```python
from build123d import *

# Parameters (mm, degrees)
SKETCH1_R           = 250
BOSS_EXTRUDE1_DEPTH = 5
SKETCH5_OUTSIDE_W   = 643.424
SKETCH5_OUTSIDE_H   = 643.424
CUT_EXTRUDE4_DEPTH  = 6
SKETCH6_R           = 2
CUT_EXTRUDE5_DEPTH  = 346.046056454
CUT_EXTRUDE6_DEPTH  = 346.046056454
SKETCH8_W           = 94.99
SKETCH8_H           = 32
CUT_EXTRUDE7_DEPTH  = 346.046056454
CUT_EXTRUDE8_DEPTH  = 346.046056454
FILLET1_R           = 2


with BuildPart() as part:
    # Sketch1 → Boss-Extrude1 (new body)
    with BuildSketch(Plane(origin=(0, 0, 0), x_dir=(1, 0, 0), z_dir=(0, 1, 0))):
        with Locations(Location((0, 0, 0), (0, 0, 270))):
            Circle(SKETCH1_R)
    extrude(amount=BOSS_EXTRUDE1_DEPTH)

    # Sketch5 outside → Cut-Extrude4 (cut)
    with BuildSketch(Plane(origin=(0, 5, 0), x_dir=(1, 0, 0), z_dir=(0, 1, 0))):
        Rectangle(SKETCH5_OUTSIDE_W, SKETCH5_OUTSIDE_H)
        Polygon((-139.754248594, -192.355221073), (139.754248594, -192.355221073), (202.254248594, -146.946313073), (250, 0), (202.254248594, 146.946313073), (77.254248594, 237.764129074), (-77.254248594, 237.764129074), (-202.254248594, 146.946313073), (-250, 0), (-202.254248594, -146.946313073), align=None, mode=Mode.SUBTRACT)
    extrude(amount=-CUT_EXTRUDE4_DEPTH, mode=Mode.SUBTRACT)

    # Sketch6 → Cut-Extrude5 (cut, through all)
    with BuildSketch(Plane.XZ):
        with Locations(Location((-3.899248594, 181.855221073, 0), (0, 0, 270))):
            Circle(SKETCH6_R)
        with Locations(Location((-199.656287114, 120.963302587, 0), (0, 0, 270))):
            Circle(SKETCH6_R)
        with Locations(Location((-232.625774638, -19.493653604, 0), (0, 0, 270))):
            Circle(SKETCH6_R)
        with Locations(Location((-176.74012291, -152.504696683, 0), (0, 0, 270))):
            Circle(SKETCH6_R)
        with Locations(Location((-53.345751406, -227.264129074, 0), (0, 0, 270))):
            Circle(SKETCH6_R)
        with Locations(Location((90.424883979, -215.216388582, 0), (0, 0, 270))):
            Circle(SKETCH6_R)
        with Locations(Location((199.656287114, -120.963302587, 0), (0, 0, 270))):
            Circle(SKETCH6_R)
        with Locations(Location((232.625774638, 19.493653604, 0), (0, 0, 270))):
            Circle(SKETCH6_R)
    extrude(amount=-CUT_EXTRUDE5_DEPTH, mode=Mode.SUBTRACT)

    # Sketch7 → Cut-Extrude6 (cut, through all)
    with BuildSketch(Plane(origin=(0, 5, 0), x_dir=(1, 0, 0), z_dir=(0, 1, 0))):
        with BuildLine():
            Line((98, 160), (98, 60))
            ThreePointArc((98, 60), (100, 58), (102, 60))
            Line((102, 60), (102, 160))
            ThreePointArc((102, 160), (100, 162), (98, 160))
        make_face()
        with BuildLine():
            Line((-48, -50), (-48, 50))
            ThreePointArc((-48, 50), (-50, 52), (-52, 50))
            Line((-52, 50), (-52, -50))
            ThreePointArc((-52, -50), (-50, -52), (-48, -50))
        make_face()
        with BuildLine():
            Line((52, -50), (52, 50))
            ThreePointArc((52, 50), (50, 52), (48, 50))
            Line((48, 50), (48, -50))
            ThreePointArc((48, -50), (50, -52), (52, -50))
        make_face()
        with BuildLine():
            Line((102, -135), (102, -60))
            ThreePointArc((102, -60), (100, -58), (98, -60))
            Line((98, -60), (98, -135))
            ThreePointArc((98, -135), (100, -137), (102, -135))
        make_face()
        with BuildLine():
            Line((-98, -135), (-98, -60))
            ThreePointArc((-98, -60), (-100, -58), (-102, -60))
            Line((-102, -60), (-102, -135))
            ThreePointArc((-102, -135), (-100, -137), (-98, -135))
        make_face()
        with BuildLine():
            Line((-98, 60), (-98, 160))
            ThreePointArc((-98, 160), (-100, 162), (-102, 160))
            Line((-102, 160), (-102, 60))
            ThreePointArc((-102, 60), (-100, 58), (-98, 60))
        make_face()
    extrude(amount=-CUT_EXTRUDE6_DEPTH, mode=Mode.SUBTRACT)

    # Sketch8 → Cut-Extrude7 (cut, through all)
    with BuildSketch(Plane.XZ):
        with Locations((0.000751406, -221.764129074)):
            Rectangle(SKETCH8_W, SKETCH8_H)
    extrude(amount=-CUT_EXTRUDE7_DEPTH, mode=Mode.SUBTRACT)

    # Sketch9 → Cut-Extrude8 (cut, through all)
    with BuildSketch(Plane(origin=(0, 5, 0), x_dir=(1, 0, 0), z_dir=(0, 1, 0))):
        Polygon((-108.026447281, -14.820317486), (-214.211563551, -14.820317486), (-174.39449797, -137.364644721), align=None)
        Polygon((-173.702637163, 137.737098208), (-213.582337829, 15), (-108.026447281, 15), align=None)
        Polygon((-70, 185.764129074), (-44.333333333, 130.764129074), (44.333333333, 130.764129074), (70, 185.764129074), align=None)
        Polygon((-35, 110.764129074), (0, 35.764129074), (35, 110.764129074), align=None)
        Polygon((0, -32.355221073), (-35, -97.355221073), (35, -97.355221073), align=None)
        Polygon((-44.333333333, -114.688554407), (-70, -162.355221073), (70, -162.355221073), (44.333333333, -114.688554407), align=None)
        Polygon((213.640720217, -14.820317486), (107.9302998, -14.820317486), (173.702637163, -137.737098208), align=None)
        Polygon((174.39449797, 137.364644721), (107.9302998, 14.64278736), (213.640720217, 16.577192616), align=None)
    extrude(amount=-CUT_EXTRUDE8_DEPTH, mode=Mode.SUBTRACT)

    # Fillet1
    fillet1_edges = [part.edges().sort_by_distance(p)[0] for p in [
        (-108.026447281, 2.5, 14.820317486),
        (-174.39449797, 2.5, 137.364644721),
        (-214.211563551, 2.5, 14.820317486),
        (-108.026447281, 2.5, -15),
        (-213.582337829, 2.5, -15),
        (-173.702637163, 2.5, -137.737098208),
        (-44.333333333, 2.5, -130.764129074),
        (-70, 2.5, -185.764129074),
        (70, 2.5, -185.764129074),
        (44.333333333, 2.5, -130.764129074),
        (-35, 2.5, -110.764129074),
        (35, 2.5, -110.764129074),
        (0, 2.5, -35.764129074),
        (-35, 2.5, 97.355221073),
        (0, 2.5, 32.355221073),
        (35, 2.5, 97.355221073),
        (-44.333333333, 2.5, 114.688554407),
        (44.333333333, 2.5, 114.688554407),
        (70, 2.5, 162.355221073),
        (-70, 2.5, 162.355221073),
        (107.9302998, 2.5, 14.820317486),
        (213.640720217, 2.5, 14.820317486),
        (173.702637163, 2.5, 137.737098208),
        (213.640720217, 2.5, -16.577192616),
        (107.9302998, 2.5, -14.64278736),
        (174.39449797, 2.5, -137.364644721),
    ]]
    fillet(fillet1_edges, radius=FILLET1_R)


solid = part.part
```
Read the model definition and answer for the solid it produces. Units are mm, in the model's axes. A direction names the side the tool comes from. Give positions to 0.01 mm unless a question says otherwise; leave off trailing zeros. Loops run counter-clockwise (first coordinate to the right, second up) from the corner with the lowest first, then second, coordinate; pieces in that order, holes last.
Item 1: Each of these flat-tipped pins is pushed along its axis until it touches: pin 1 Ø1.5 at (y, z) = (2, 112) entering from -X; pin 2 Ø1.5 at (x, y) = (-3, 2.5) entering from -Z; pin 3 Ø2.5 at (y, z) = (2, -215.5) entering from -X. Where does it stop, or does it pass through?
Item 2: For faces 1 (the flat face through (-141.34, 2.54, 76.33)), 2 (the flat face through (-171.442, 2.535, 169.333)), determine the directions among +Z, -Z, +X, -X, +Y, -Y from which every point of the face is accessible in a straight line to the end or side of a thin tool.
Item 3: The mould has two halves that part along Z. Classify faces 3 (the flat face through (56.82, 2.54, 137.88)), 4 (the flat face through (226.461, 2.535, -72.445)), 5 (the flat face through (170.567, 2.535, 169.969)): released by +Z, released by -Z, zero draft, split by the parting line, or undercut.
Item 4: The part is cut by section A-A (x = -189). Write down the section's boundary in (y, z), and give its area (3 significant figures).
Item 5: The part is cut by section C-C (x = 124). Write down the section's boundary in (y, z), and give its area (3 significant figures).
Item 6: Find the intervals of material crossed by line 1 along X through (y, z) = (2.1, 3); line 2 along X through (y, z) = (3.05, -217); line 3 along Z through (x, y) = (-19.5, 3.1), in increasing order.
Item 7: The part is cut by section B-B (y = 1.25). Give the number of separate pieces and of enclosed holes in the cut face, and give its area (3 significant figures).
Taken from the geometry:
1. pin 1: stops at x = -213.85
1. pin 2: stops at z = -205.76
1. pin 3: stops at x = -109.62
2. face 1: +Y, -Y
2. face 2: +Z, -X, +Y, -Y
3. face 3: undercut
3. face 4: released by -Z
3. face 5: released by +Z
4. outline: (0, -156.58) - (5, -156.58) - (5, -90.66) - (0, -90.66) - close; (0, -15) - (5, -15) - (5, 14.82) - (0, 14.82) - close; (0, 92.41) - (5, 92.41) - (5, 156.58) - (0, 156.58) - close
4. area: 800 mm2
5. outline: (0, -203.8) - (5, -203.8) - (5, -44.31) - (0, -44.31) - close; (0, -14.94) - (5, -14.94) - (5, 14.82) - (0, 14.82) - close; (0, 44.85) - (5, 44.85) - (5, 192.36) - (0, 192.36) - close
5. area: 1,680 mm2
6. line 1: x = -249.03 to -52, -48 to 48, 52 to 249.03
6. line 2: x = -105.83 to -47.49, 47.5 to 89.52, 91.33 to 105.83
6. line 3: z = -205.76 to -185.76, -130.76 to -110.76, -77.55 to 68.57, 97.36 to 114.69, 162.36 to 192.36
7. separate pieces: 1
7. enclosed holes: 22
7. area: 126,000 mm2
